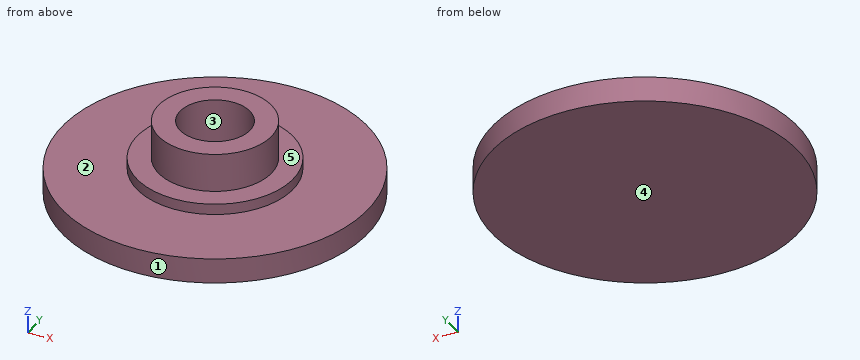
```python
from build123d import *

# Parameters (mm, degrees)
F0_W = 1.524
F0_H = 0.762


with BuildPart() as f1:
    # F0 (on Front) → F1 (revolve)
    with BuildSketch(Plane.XZ):
        Polygon((0, 1.778), (0, 0), (10.795, 0), (10.795, 1.778), (5.5245, 1.778), (4.0005, 1.778), (4.0005, 2.54), (4.0005, 5.2705), (2.4765, 5.2705), (2.4765, 1.778), align=None)
        with Locations((4.7625, 2.159)):
            Rectangle(F0_W, F0_H)
    revolve(axis=Axis((0, 0, 13.315846), (0, 0, -1)))


solid = f1.part
```
Geometry: final body of the model. Coordinates: model frame, mm. Face numbers are marked on the shaded views. A direction names the side the tool comes from. Give positions to 0.01 mm unless a question says otherwise; leave off trailing zeros. Order: outer loops, then holes, each group sorted by start corner. A loop starts at its lowest first (then second) coordinate and runs counter-clockwise, first axis right, second up. Notation, with made-up numbers: M 37.25,81 L 94.25,81 A14 ccw 94.25,101 Z; hole C 78,-7 d2. An arc over 180 degrees is marked long. Answer as CSV lines item,"result". Start each with the question number.
1) First-contact query: P1, Ø6, axis at x = 4.5, y = 3.5, coming from the -Z side; P2, Ø1.5, axis at x = 6.5, z = 4.5, coming from the -Y side; P3, Ø1, axis at x = 1.5, z = 3.5, coming from the +Y side; P4, Ø2, axis at x = -4, z = 4, coming from the +Y side. Flat tips, straight axial feed; report the tip coordinate or a pass-through.
2) Mould query, pull axis X, two halves, no side actions, for the marked faces 1, 2 and 3. Classes: +X half, -X half, draft (parallel to the pull), parting line (faces both ways), or undercut.
3) Line query: line 1 (X direction, y = 0, z = 2.85); line 2 (Z direction, x = -1.25, y = -9.5). Output: solid intervals per line, ascending. Write a range as from..to.
4) Cut plane D-D (y = -4.5). Output: boundary loops of the cut face in (x, z).
5) Cut plane A-A (x = 0). Output: boundary loops of the cut face in (y, z) (1 decimal).
6) Set-up query: the marked faces 4 and 5. Return all of +Z, -Z, +X, -X, +Y, -Y with unobstructed straight access to the full face (end or side cutting, diameter ignored); none if empty.
7) Cut plane C-C (z = 3.35). Output: boundary loops of the cut face in (x, y).
Findings below:
1,P1,"stops at z = 0"
1,P2,"passes through"
1,P3,"stops at y = 3.87"
1,P4,"stops at y = 2.65"
2,face 1,"parting line"
2,face 2,"draft"
2,face 3,"undercut"
3,line 1,"x = -4..-2.48, 2.48..4"
3,line 2,"z = 0..1.78"
4,outline,"M -9.81,0 L 9.81,0 L 9.81,1.78 L 3.2,1.78 L 3.2,2.54 L -3.2,2.54 L -3.2,1.78 L -9.81,1.78 Z"
5,outline,"M -10.8,0 L 10.8,0 L 10.8,1.8 L 5.5,1.8 L 5.5,2.5 L 4,2.5 L 4,5.3 L 2.5,5.3 L 2.5,1.8 L -2.5,1.8 L -2.5,5.3 L -4,5.3 L -4,2.5 L -5.5,2.5 L -5.5,1.8 L -10.8,1.8 Z"
6,face 4,"-Z, +X, -X, +Y, -Y"
6,face 5,"+Z"
7,outline,"C 0,0 d8; hole C 0,0 d4.95"
